Autodesk Inventor part; units mm, degrees
ref_plane "YZ Plane" through (0, 0, 0) normal (1, 0, 0) x (0, 1, 0)
ref_plane "XZ Plane" through (0, 0, 0) normal (0, 1, 0) x (-1, 0, 0)
ref_plane "XY Plane" through (0, 0, 0) normal (0, 0, 1) x (1, 0, 0)
sketch "スケッチ1" plane through (0, 0, 0) normal (0, 0, 1) x (1, 0, 0)
  line L0 (0, 0) -> (0, -111.3423) construction
  line L1 (-42.5, 0) -> (-47.5, 0)
  line L2 (-47.5, 0) -> (-47.5, -105)
  line L3 (-47.5, -105) -> (-42.5, -105)
  line L4 (-42.5, -105) -> (-42.5, 0)
  dimension "d0" = 105
  dimension "d1" = 5
  dimension "d2" = 47.5
revolve "回転1" add sketch "スケッチ1" angle 360 about axis through (0, 0, 0) along (0, -1, 0)
sketch "スケッチ2" plane through (0, 0, 0) normal (0, 1, 0) x (1, 0, 0)
  circle A0 centre (0, 0) radius 42.5
  line L0 (100, 100) -> (-100, 100)
  line L1 (-100, 100) -> (-100, -100)
  line L2 (-100, -100) -> (100, -100)
  line L3 (100, -100) -> (100, 100)
  line L4 (100, 100) -> (-100, -100) construction
  line L5 (-100, 100) -> (100, -100) construction
  circle A1 centre (80, -80) radius 4
  circle A2 centre (80, 80) radius 4
  circle A3 centre (-80, 80) radius 4
  circle A4 centre (-80, -80) radius 4
  dimension "d4" = 200
  dimension "d7" = 8
  dimension "d8" = 20
  dimension "d11" = 360
extrude "押し出し1" add sketch "スケッチ2" against normal blind 5 contours A0 | L3 L2 L1 L0
sketch "スケッチ3" plane through (0, 0, 0) normal (0, 0, 1) x (1, 0, 0)
  circle A0 centre (0, -25) radius 6
  line L0 (42.5, -5) -> (-42.5, -5)
  point P0 (0, 0)
  dimension "d13" = 12
  dimension "d14" = 20
extrude "押し出し2" cut sketch "スケッチ3" along normal through all both and the other way through all
properties part number "Wind Trubin Turbine Base"
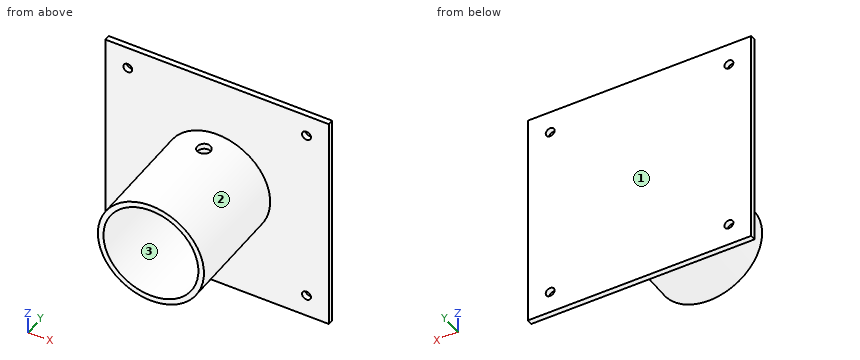
Geometry: final body of the model. Coordinates: model frame, mm. Face numbers are marked on the shaded views. Coordinates: 2 decimals unless noted, no trailing zeros. Order: outer loops, then holes, each group sorted by start corner. A loop starts at its lowest first (then second) coordinate and runs counter-clockwise, first axis right, second up.
Item 1: Draft query along Z for the marked faces 1, 2 and 3. Return one class per face: released by +Z, released by -Z, zero draft, split by the parting line, or undercut.
Answer:
face 1: zero draft
face 2: split by the parting line
face 3: undercut
Item 2: Section query B-B (x = 80). Output: boundary loops of the cut face in (y, z).
Answer:
outline: (-5, -100) - (0, -100) - (0, -84) - (-5, -84) - close; (-5, -76) - (0, -76) - (0, 76) - (-5, 76) - close; (-5, 84) - (0, 84) - (0, 100) - (-5, 100) - close
Item 3: Contact query for flat-ended pins moving along their axis: P1, Ø4, axis at x = 49.5, z = 56, coming from the -Y side; P2, Ø1.5, axis at y = -28.5, z = -22.5, coming from the -X side; P3, Ø7, axis at x = -80, z = -80, coming from the +Y side; P4, Ø14, axis at x = 0, y = -25, coming from the -Z side. Output: stop coordinate, or through.
Answer:
P1: stops at y = -5
P2: stops at x = -42.23
P3: passes through
P4: stops at z = -47.5
Item 4: Section query C-C (y = -74). Output: boundary loops of the cut face in (x, z).
Answer:
outline: circle Ø95 at (0, 0); hole circle Ø85 at (0, 0)
Item 5: Section query D-D (z = 0). Output: boundary loops of the cut face in (x, y), then the cut area to 3 significant figures.
Answer:
outline: (-100, -5) - (-47.5, -5) - (-47.5, -105) - (-42.5, -105) - (-42.5, -5) - (42.5, -5) - (42.5, -105) - (47.5, -105) - (47.5, -5) - (100, -5) - (100, 0) - (-100, 0) - close
area: 2,000 mm2
Item 6: Section query A-A (z = 80). Output: boundary loops of the cut face in (x, y).
Answer:
outline: (-100, -5) - (-84, -5) - (-84, 0) - (-100, 0) - close; (-76, -5) - (76, -5) - (76, 0) - (-76, 0) - close; (84, -5) - (100, -5) - (100, 0) - (84, 0) - close
Item 7: Material intervals for line 1 along X through (y, z) = (-2.6, -80); line 2 along Y through (x, z) = (0, -44.1), sorted ascending.
Answer:
line 1: x = -100 to -84, -76 to 76, 84 to 100
line 2: y = -105 to -31, -19 to 0
